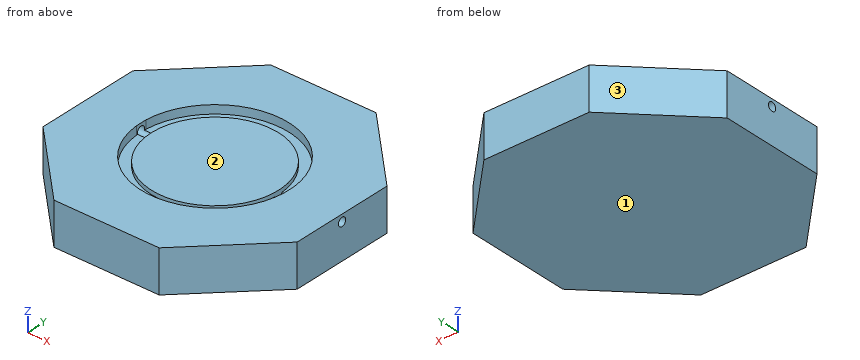
```python
from build123d import *

# Parameters (mm, degrees)
F1_DEPTH       = 40
F2_R           = 22.5
F3_DEPTH       = 3
F5_DEPTH       = 25
F6_DEPTH       = 25
F7_DEPTH       = 25
F8_R           = 1.5
F9_DEPTH       = 110
F10_END_RADIUS = 22.5
F10_REACH      = 49.2436407871
F11_END_RADIUS = 22.5
F11_REACH      = 49.2436407871
F12_DEPTH      = 1.6


with BuildPart() as f1:
    # F0 (on Top) → F1 (new body)
    with BuildSketch(Plane.XY):
        Polygon((18.6396103068, 45), (-18.6396103068, 45), (-45, 18.6396103068), (-45, -18.6396103068), (-18.6396103068, -45), (18.6396103068, -45), (45, -18.6396103068), (45, 18.6396103068), align=None)
    extrude(amount=F1_DEPTH)

    # F2 (on face) → F3 (cut)
    with BuildSketch(Plane.XY.offset(40)):
        with BuildLine():
            Line((-26.1736986305, 2), (-26.1736986305, -2))
            ThreePointArc((-26.1736986305, -2), (0, -26.25), (26.1736986305, -2))
            Line((26.1736986305, -2), (26.1736986305, 2))
            ThreePointArc((26.1736986305, 2), (0, 26.25), (-26.1736986305, 2))
        make_face()
        Circle(F2_R, mode=Mode.SUBTRACT)
    extrude(amount=-F3_DEPTH, mode=Mode.SUBTRACT)

    # F4 (on face) → F5 (join)
    with BuildSketch(Plane.XY):
        Polygon((-18.6396103068, -45), (18.6396103068, -45), (45, -18.6396103068), (45, 18.6396103068), (18.6396103068, 45), (-18.6396103068, 45), (-45, 18.6396103068), (-45, -18.6396103068), align=None)
    extrude(amount=F5_DEPTH)

    # F0 (on Top) → F6 (join)
    with BuildSketch(Plane.XY):
        Polygon((18.6396103068, 45), (-18.6396103068, 45), (-45, 18.6396103068), (-45, -18.6396103068), (-18.6396103068, -45), (18.6396103068, -45), (45, -18.6396103068), (45, 18.6396103068), align=None)
    extrude(amount=F6_DEPTH)

    # F0 (on Top) → F7 (cut)
    with BuildSketch(Plane.XY):
        Polygon((18.6396103068, 45), (-18.6396103068, 45), (-45, 18.6396103068), (-45, -18.6396103068), (-18.6396103068, -45), (18.6396103068, -45), (45, -18.6396103068), (45, 18.6396103068), align=None)
    extrude(amount=F7_DEPTH, mode=Mode.SUBTRACT)

    # F8 (on Right) → F9 (cut, symmetric)
    with BuildSketch(Plane.YZ):
        with Locations((0, 37.5)):
            Circle(F8_R)
    extrude(amount=F9_DEPTH, both=True, mode=Mode.SUBTRACT)

    f10_end = (Plane.XY.offset(38.5) * Cylinder(F10_END_RADIUS, 354.8073942381, mode=Mode.PRIVATE)).faces().sort_by_distance((-22.5, 0, 39.3628971796))[0]
    # F8 (on Right) → F10 (join, up to the whole of a round face its end follows)
    with BuildSketch(Plane.YZ):
        with Locations((0, 37.5)):
            Circle(F8_R)
    f10_long = extrude(amount=F10_REACH, mode=Mode.PRIVATE)
    add(split(f10_long, bisect_by=f10_end, keep=Keep.BOTTOM, mode=Mode.PRIVATE))

    f11_end = (Plane.XY.offset(38.5) * Cylinder(F11_END_RADIUS, 354.8073942381, mode=Mode.PRIVATE)).faces().sort_by_distance((-22.5, 0, 39.3628971796))[0]
    # F8 (on Right) → F11 (join, up to the whole of a round face its end follows)
    with BuildSketch(Plane.YZ):
        with Locations((0, 37.5)):
            Circle(F8_R)
    f11_long = extrude(amount=-F11_REACH, mode=Mode.PRIVATE)
    add(split(f11_long, bisect_by=f11_end, keep=Keep.BOTTOM, mode=Mode.PRIVATE))

    # F12 (cut): a face of the model
    f12_faces = [f1.faces().sort_by_distance(p)[0] for p in [
        (0, 0, 40),
    ]]
    extrude(f12_faces, amount=-F12_DEPTH, mode=Mode.SUBTRACT)


solid = f1.part
```
Could you check a few things on this model? Use its own coordinates, in mm. Face numbers are marked on the shaded views. Round coordinates to 2 decimals unless told otherwise and drop trailing zeros. Write each loop counter-clockwise with the first axis right and the second up, starting at its lowest first coordinate (ties: lowest second). Pieces come first, ordered by that corner, then holes. Notation, with made-up numbers: M -13,79.25 L 27,79.25 A7 cw 27,86.25 Z; hole C -34.75,39.5 d5. An arc over 180 degrees is marked long. Answer in a Markdown table with one row per item. Add a question column.
Q1. Will these pins go through, and if not, where does the flat tip stop? pin 1 Ø7.5 at (x, y) = (-9.5, -9) entering from +Z; pin 2 Ø3 at (x, z) = (23.5, 30) entering from -Y; pin 3 Ø1.5 at (y, z) = (28, 28) entering from -X.
Q2. Imagine slicing it at A-A (y = 0). Please give me the cut outline in (x, z).
Q3. If we mould it in two halves opening along X, with no side actions, what happens to the marked faces 1, 2 and 3? For each: +X half, -X half, draft (parallel to the pull), parting line (faces both ways), or undercut.
Q4. Imagine slicing it at C-C (z = 33.75). Please give me the cut outline in (x, y).
Q5. If I drill on line 1 (Z direction, x = -30, y = 0); line 2 (Z direction, x = 1.5, y = -21); line 3 (Y direction, x = -28.25, z = 37.5), over which ranges is the centre line in solid material (lowest first)? Write a range as from..to.
Q6. Imagine slicing it at B-B (x = 0). Please give me the cut outline in (y, z), then the cut area to 3 significant figures.
Q7. Imagine slicing it at D-D (y = 16). Please give me the cut outline in (x, z), then the cut area to 3 significant figures.
Values:
| question | item | result |
|---|---|---|
| 1 | pin 1 | z = 38.4 |
| 1 | pin 2 | y = -41.64 |
| 1 | pin 3 | x = -36.39 |
| 2 | outline | M -45,25 L 45,25 L 45,36 L 22.5,36 L 22.5,38.4 L -22.5,38.4 L -22.5,36 L -45,36 Z; M -45,39 L -26.17,39 L -26.17,40 L -45,40 Z; M 26.17,39 L 45,39 L 45,40 L 26.17,40 Z |
| 3 | face 1 | draft |
| 3 | face 2 | undercut |
| 3 | face 3 | -X half |
| 4 | outline | M -45,-18.64 L -18.64,-45 L 18.64,-45 L 45,-18.64 L 45,18.64 L 18.64,45 L -18.64,45 L -45,18.64 Z |
| 5 | line 1 | 25..36, 39..40 |
| 5 | line 2 | 25..38.4 |
| 5 | line 3 | -35.39..-1.5, 1.5..35.39 |
| 6 | outline | M -45,25 L 45,25 L 45,40 L 26.25,40 L 26.25,37 L 22.5,37 L 22.5,38.4 L -22.5,38.4 L -22.5,37 L -26.25,37 L -26.25,40 L -45,40 Z |
| 6 | area | 1,260 mm^2 |
| 7 | outline | M -45,25 L 45,25 L 45,40 L 20.81,40 L 20.81,37 L 15.82,37 L 15.82,38.4 L -15.82,38.4 L -15.82,37 L -20.81,37 L -20.81,40 L -45,40 Z |
| 7 | area | 1,270 mm^2 |
